CAD build for the part. Positions are in the model's coordinates, mm. Round coordinates to 2 decimals unless told otherwise and drop trailing zeros. Loops run counter-clockwise (first coordinate to the right, second up) from the corner with the lowest first, then second, coordinate; pieces in that order, holes last.
from build123d import *

# Parameters (mm, degrees)
SKETCH_2_R      = 60
SKETCH_2_R_2    = 50
EXTRUDE_2_DEPTH = 3
M3_HUB_BOARD_D  = 3.6


with BuildPart() as part:
    # ｽｹｯﾁ2 → ﾎﾞｽ - 押し出し2 (new body)
    with BuildSketch(Plane(origin=(0, 0, 0), x_dir=(1, 0, 0), z_dir=(0, 1, 0))):
        with Locations(Location((0, 0, 0), (0, 0, 270))):
            Circle(SKETCH_2_R)
        with Locations(Location((0, 0, 0), (0, 0, 270))):
            Circle(SKETCH_2_R_2, mode=Mode.SUBTRACT)
    extrude(amount=EXTRUDE_2_DEPTH)

    # M3 Hub_Boardへの固定用穴 (through all)
    with Locations(Plane(origin=(-31.622776602, 3, -45), x_dir=(0, 0, 1), z_dir=(0, 1, 0))):
        with Locations((0, 0), (0, 63.245553204)):
            m3_hub_board = Hole(M3_HUB_BOARD_D / 2)

    # ﾐﾗｰ1: M3 Hub_Boardへの固定用穴 across plane
    add(m3_hub_board.mirror(Plane.XY), mode=Mode.SUBTRACT)


solid = part.part
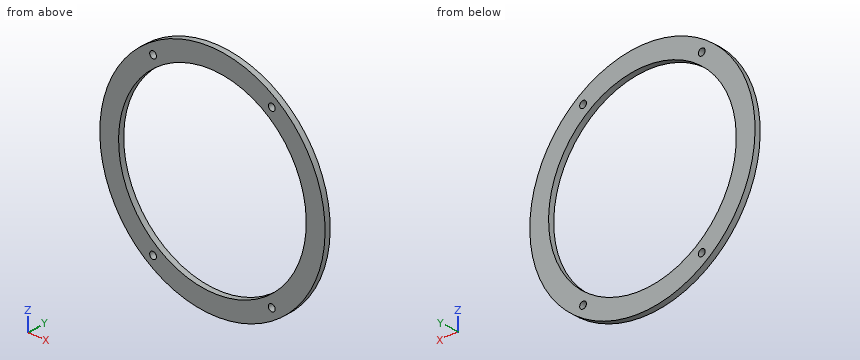
Item 1: Flat gauge pins, fed straight in: P1, Ø1, axis at x = 43.5, y = 0.5, coming from the -Z side; P2, Ø3, axis at x = 31.62, z = 45, coming from the -Y side. Where does each tip first touch, or does it go through?
Verdict:
P1: stops at z = -41.84
P2: passes through
Item 2: Cut at B-B (x = 0). List the corners of the cut face in (y, z), plus the area to 3 significant figures.
Verdict:
outline: (0, -60) - (3, -60) - (3, -50) - (0, -50) - close; (0, 50) - (3, 50) - (3, 60) - (0, 60) - close
area: 60.0 mm2
Item 3: Wall check: L1, parallel to X at y = 1.3, z = 0; L2, parallel to Z at x = 33, y = 0.3; L3, parallel to X at y = 2.35, z = 44. Give the ranges that are in metal, low to high.
Verdict:
L1: x = -60 to -50, 50 to 60
L2: z = -50.11 to -46.16, -43.84 to -37.56, 37.56 to 43.84, 46.16 to 50.11
L3: x = -40.79 to -33.12, -30.13 to -23.75, 23.75 to 30.13, 33.12 to 40.79
Item 4: Cut at C-C (z = -45). List the corners of the cut face in (x, y).
Verdict:
outline: (-39.69, 0) - (-33.42, 0) - (-33.42, 3) - (-39.69, 3) - close; (-29.82, 0) - (-21.79, 0) - (-21.79, 3) - (-29.82, 3) - close; (21.79, 0) - (29.82, 0) - (29.82, 3) - (21.79, 3) - close; (33.42, 0) - (39.69, 0) - (39.69, 3) - (33.42, 3) - close
Item 5: Cut at A-A (z = 0). List the corners of the cut face in (x, y), plus the area to 3 significant figures.
Verdict:
outline: (-60, 0) - (-50, 0) - (-50, 3) - (-60, 3) - close; (50, 0) - (60, 0) - (60, 3) - (50, 3) - close
area: 60.0 mm2
Item 6: Cut at D-D (y = 2). List the corners of the cut face in (x, z).
Verdict:
outline: circle Ø120 at (0, 0); hole circle Ø100 at (0, 0); hole circle Ø3.6 at (-31.62, -45); hole circle Ø3.6 at (-31.62, 45); hole circle Ø3.6 at (31.62, -45); hole circle Ø3.6 at (31.62, 45)
